Geometry check sheet. Reference: the model listing, model coordinates, mm. A direction names the side the tool comes from. Round coordinates to 2 decimals unless told otherwise and drop trailing zeros. Order: outer loops, then holes, each group sorted by start corner. A loop starts at its lowest first (then second) coordinate and runs counter-clockwise, first axis right, second up. Notation, with made-up numbers: (-10.5, -7) - (18.5, -7) arc R25 cw to (18.5, 11) - close; hole circle Ø7 at (58, 35). An arc over 180 degrees is marked (long way). One line per question, with ' | ' between items. Start each with the question number.
Q1. Tool access check on faces 1 (the face through (-7.395, 104.638, -13.051)), 2 (the face through (13.45, 47.68, -7.81)), 3 (the face through (-13.49, 47.68, -7.74)), 4 (the face through (-15, 105, 0)). Record the directions out of +Z, -Z, +X, -X, +Y, -Y that give a thin tool (end or side, any length) a straight path to the whole face; none if there is none.
Q2. Sectioned sample at B-B, the plane x = 41.75. Enter the section's corners in (y, z).
Q3. Sectioned sample at A-A, the plane y = 100.5. Enter the section's corners in (x, z), then the cut area to 3 significant figures.
Q4. Mould release check, pull along X, two halves, no side actions. Record for faces 5 (the face through (-10, 37, 0)), 6 (the face through (-37.88, 5.07, 3.55)), 7 (the face through (3, 112.75, 10)): +X half, -X half, draft (parallel to the pull), parting line (faces both ways), or undercut.
Q5. Material ranges on line 1 along Z through (x, y) = (-41, 7); line 2 along Y through (x, z) = (11, 12.5); line 3 along Y through (x, z) = (-21, 21.5), recorded low to high.
Q6. Sectioned sample at D-D, the plane y = 70. Enter the section's corners in (x, z).
Q7. Gauge pin test, flat ends, axial feed: P1, Ø5, axis at y = 45, z = -4.5, coming from the +X side; P2, Ø5, axis at y = 39.5, z = -16.5, coming from the -X side; P3, Ø8, axis at x = -32, z = -24, coming from the +Y side. Record the tip position at first contact, or that the pin passes through.
Q8. Sectioned sample at C-C, the plane x = -39. Enter the section's corners in (y, z).
```python
from build123d import *

# Parameters (mm, degrees)
EXTRUDE_1_DEPTH     = 10
EXTRUDE_2_DEPTH     = 16
SKETCH_5_R          = 5.25
CUT_EXTRUDE_1_DEPTH = 11


with BuildPart() as part:
    # Эскиз1 → Повернуть1 (revolve)
    with BuildSketch(Plane.XY, mode=Mode.PRIVATE) as revolve_1_sk:
        Polygon((0, 0), (-50, 0), (-50, 10), (-30, 10), (-22, 29), (-15, 29), (-15, 31), (-10, 36), (-10, 38), (-10, 48), (-10, 145.5), (-7.5, 148), (0, 148), align=None)
    revolve(revolve_1_sk.sketch.rotate(Axis((0, 0, 0), (0, 1, 0)), 180), axis=Axis((0, 0, 0), (0, 1, 0)))  # turned: the seam where the file's is

    # Эскиз2 → Бобышка-Вытянуть1 (add)
    with BuildSketch(Plane(origin=(0, 38, 0), x_dir=(1, 0, 0), z_dir=(0, 1, 0))):
        Polygon((0, 17.320508076), (-15, 8.660254038), (-15, -8.660254038), (0, -17.320508076), (15, -8.660254038), (15, 8.660254038), align=None)
    extrude(amount=EXTRUDE_1_DEPTH)

    # Эскиз3 → Бобышка-Вытянуть2 (add)
    with BuildSketch(Plane(origin=(0, 96.75, 0), x_dir=(1, 0, 0), z_dir=(0, 1, 0))):
        Polygon((15, 8.660254038), (0, 17.320508076), (-15, 8.660254038), (-15, -8.660254038), (0, -17.320508076), (15, -8.660254038), align=None)
    extrude(amount=EXTRUDE_2_DEPTH)

    # Эскиз4 → Вырез-Повернуть2 (revolve, cut)
    with BuildSketch(Plane.XY, mode=Mode.PRIVATE) as cut_revolve_2_sk:
        Polygon((-28.856406461, 112.75), (-15, 112.75), (-28.856406461, 104.75), align=None)
        Polygon((-28.856406461, 96.75), (-28.856406461, 104.75), (-15, 96.75), align=None)
        Polygon((-23.660254038, 48), (-23.660254038, 43), (-15, 48), align=None)
        Polygon((-23.660254038, 43), (-23.660254038, 38), (-15, 38), align=None)
    revolve(cut_revolve_2_sk.sketch.rotate(Axis((0, 148, 0), (0, -1, 0)), 180), axis=Axis((0, 148, 0), (0, -1, 0)), mode=Mode.SUBTRACT)  # turned: the seam where the file's is

    # Эскиз5 → Вырез-Вытянуть1 (cut, through all)
    with BuildSketch(Plane(origin=(0, 10, 0), x_dir=(1, 0, 0), z_dir=(0, 1, 0))):
        with Locations(Location((-41.75, 0, 0), (0, 0, 180))):  # turned: the seam where the file's is
            Circle(SKETCH_5_R)
        with Locations(Location((41.75, 0, 0), (0, 0, 180))):  # turned: the seam where the file's is
            Circle(SKETCH_5_R)
    extrude(amount=-CUT_EXTRUDE_1_DEPTH, mode=Mode.SUBTRACT)


solid = part.part
```
Determined:
1) face 1: -Z, -X, +Y | face 2: -Z, +X | face 3: -Z, -X | face 4: +Z, -Z, -X, +Y
2) outline: (0, -27.51) - (10, -27.51) - (10, -5.25) - (0, -5.25) - close; (0, 5.25) - (10, 5.25) - (10, 27.51) - (0, 27.51) - close
3) outline: (-15, -8.66) - (0, -17.32) - (15, -8.66) - (15, 8.66) - (0, 17.32) - (-15, 8.66) - close | area: 779 mm2
4) face 5: parting line | face 6: undercut | face 7: draft
5) line 1: z = -28.62 to -5.2, 5.2 to 28.62 | line 2: y = 0 to 29 | line 3: y = 0 to 10
6) outline: circle Ø20 at (0, 0)
7) P1: stops at x = 15 | P2: stops at x = -5.75 | P3: stops at y = 10
8) outline: (0, -31.29) - (10, -31.29) - (10, -4.47) - (0, -4.47) - close; (0, 4.47) - (10, 4.47) - (10, 31.29) - (0, 31.29) - close
